Check sheet for the drawn part. Datum: minimum x, y, z corner. Units: mm. A direction names the side the tool comes from. Give positions to 0.01 mm unless a question says otherwise; leave off trailing zeros. Order: outer loops, then holes, each group sorted by start corner. A loop starts at its lowest first (then second) coordinate and runs counter-clockwise, first axis right, second up. Notation, with made-up numbers: (34, 43.5) - (77, 43.5) arc R17 cw to (77, 57.5) - close; hole circle Ø2 at (48, -25). An arc over 180 degrees is marked (long way). Answer as a JSON object with one key per item and string values. Group by question number.
(1) Depth check by flat-ended pin: pin 1 Ø4.5 at (x, y) = (53, 61) entering from -Z; pin 2 Ø9 at (x, y) = (24.5, 13.5) entering from +Z. Enter the tip coordinate at first touch or a pass-through.
(2) Thickness scan on line 1 (Y direction, x = 30, z = 18.75); line 2 (X direction, y = 20.5, z = 27); line 3 (Y direction, x = 7, z = 15.5). Record the ranges inside material, lowest first.
(3) Access from +Z, -Z, +X, -X, +Y, -Y to the whole of each face (thin tool, end or side, straight path). Record for the marked faces 1, 2 and 3.
(4) Section check D-D (x = 22.5). Record the boundary of the cut face in (y, z), then the cut area to 3 significant figures.
(5) Section check A-A (z = 22.5). Record the boundary of the cut face in (x, y).
(6) Section check B-B (y = 100). Record the boundary of the cut face in (x, z).
(7) Section check C-C (z = 36). Record the boundary of the cut face in (x, y).
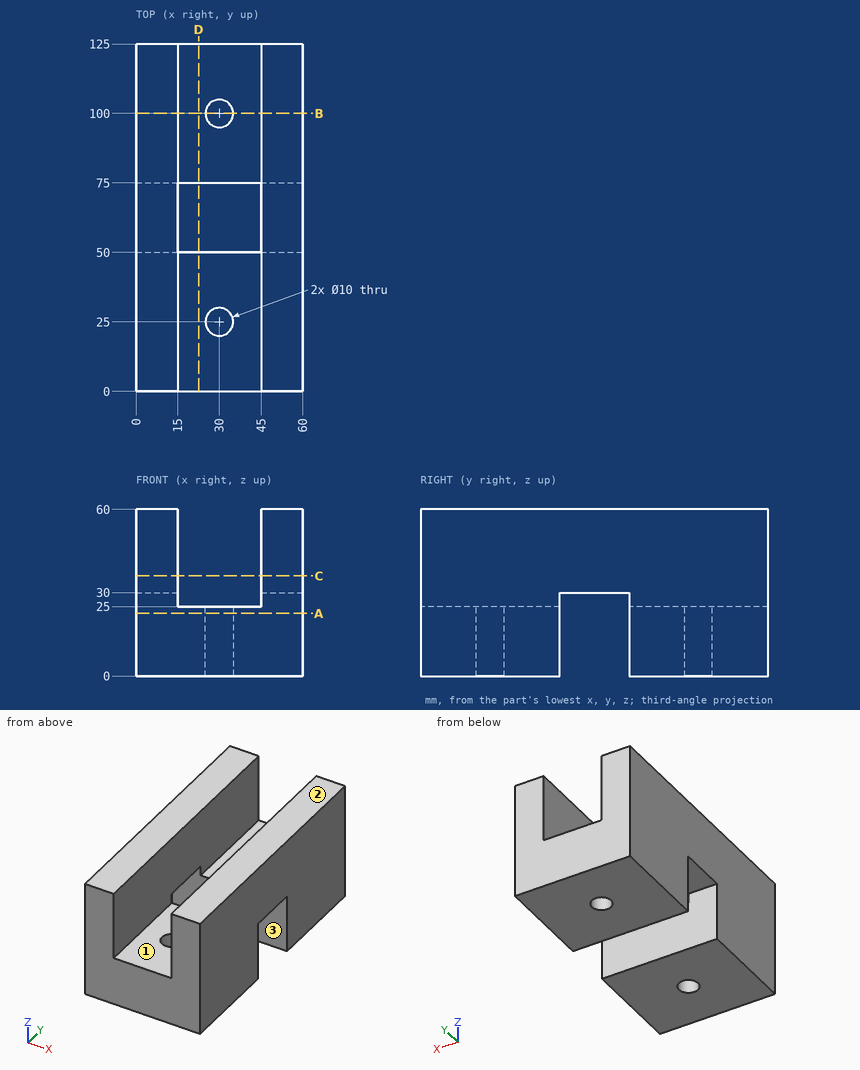
Solutions:
{
 "1": {"pin 1": "stops at z = 30", "pin 2": "stops at z = 25"},
 "2": {"line 1": "y = 0 to 20, 30 to 50, 75 to 95, 105 to 125", "line 2": "x = 0 to 15, 45 to 60", "line 3": "y = 0 to 50, 75 to 125"},
 "3": {"face 1": "+Z, +Y, -Y", "face 2": "+Z, +X, -X, +Y, -Y", "face 3": "-Z, +X, -X"},
 "4": {"outline": "(0, 0) - (50, 0) - (50, 25) - (0, 25) - close; (75, 0) - (125, 0) - (125, 25) - (75, 25) - close", "area": "2,500 mm2"},
 "5": {"outline": "(0, 0) - (60, 0) - (60, 50) - (0, 50) - close; (0, 75) - (60, 75) - (60, 125) - (0, 125) - close; hole circle Ø10 at (30, 25); hole circle Ø10 at (30, 100)"},
 "6": {"outline": "(0, 0) - (25, 0) - (25, 25) - (15, 25) - (15, 60) - (0, 60) - close; (35, 0) - (60, 0) - (60, 60) - (45, 60) - (45, 25) - (35, 25) - close"},
 "7": {"outline": "(0, 0) - (15, 0) - (15, 125) - (0, 125) - close; (45, 0) - (60, 0) - (60, 125) - (45, 125) - close"}
}
